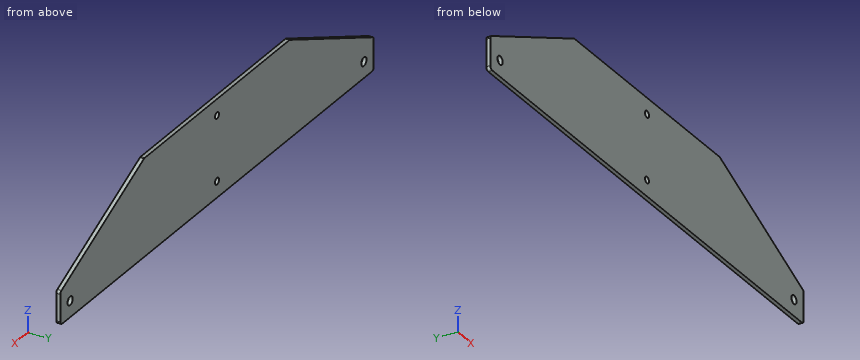
```python
from build123d import *

# Parameters (mm, degrees)
SKETCH1_W           = 406.4
SKETCH1_H           = 76.2
SKETCH1_R           = 3.3734375
SKETCH1_R_2         = 2.5796875
BOSS_EXTRUDE1_DEPTH = 3.175
CHAMFER1_SIZE       = 50.8
CHAMFER1_SIZE2      = 108.940951562
CHAMFER2_SIZE       = 50.8
CHAMFER2_SIZE2      = 108.940951562
FILLET1_R           = 2.54


with BuildPart() as part:
    # Sketch1 → Boss-Extrude1 (new body)
    with BuildSketch(Plane(origin=(0, 0, 0), x_dir=(1, 0, 0), z_dir=(0, 1, 0))):
        Rectangle(SKETCH1_W, SKETCH1_H)
        with Locations(Location((-190.5, 25.4, 0), (0, 0, 270))):
            Circle(SKETCH1_R, mode=Mode.SUBTRACT)
        with Locations(Location((190.5, 25.4, 0), (0, 0, 270))):
            Circle(SKETCH1_R, mode=Mode.SUBTRACT)
        with Locations(Location((0, 25.4, 0), (0, 0, 270))):
            Circle(SKETCH1_R_2, mode=Mode.SUBTRACT)
        with Locations(Location((0, -25.4, 0), (0, 0, 270))):
            Circle(SKETCH1_R_2, mode=Mode.SUBTRACT)
    extrude(amount=BOSS_EXTRUDE1_DEPTH)

    # Chamfer1
    chamfer1_edges = [part.edges().sort_by_distance(p)[0] for p in [
        (-203.2, 1.5875, 38.1),
    ]]
    chamfer1_side = [part.faces().sort_by_distance(p)[0] for p in [
        (-203.2, 1.5875, 0),
    ]]
    chamfer(chamfer1_edges, length=CHAMFER1_SIZE, length2=CHAMFER1_SIZE2, reference=chamfer1_side[0])

    # Chamfer2
    chamfer2_edges = [part.edges().sort_by_distance(p)[0] for p in [
        (203.2, 1.5875, 38.1),
    ]]
    chamfer2_side = [part.faces().sort_by_distance(p)[0] for p in [
        (203.2, 1.5875, 0),
    ]]
    chamfer(chamfer2_edges, length=CHAMFER2_SIZE, length2=CHAMFER2_SIZE2, reference=chamfer2_side[0])

    # Fillet1
    fillet1_edges = [part.edges().sort_by_distance(p)[0] for p in [
        (-94.259048438, 1.5875, 38.1),
        (-203.2, 1.5875, -12.7),
        (203.2, 1.5875, -12.7),
        (94.259048438, 1.5875, 38.1),
        (-203.2, 1.5875, -38.1),
        (203.2, 1.5875, -38.1),
    ]]
    fillet(fillet1_edges, radius=FILLET1_R)


solid = part.part
```
CAD build for the part. Positions are in the model's coordinates, mm. Coordinates: 2 decimals unless noted, no trailing zeros. Order: outer loops, then holes, each group sorted by start corner. A loop starts at its lowest first (then second) coordinate and runs counter-clockwise, first axis right, second up. Notation, with made-up numbers: (83, 32.25) -> (98, 32.25) arc R16 cw to (98, 54.25) -> close; hole circle Ø9 at (27.25, 51). An arc over 180 degrees is marked (long way). Use one line per item in the form item = value. Start each with the question number.
1) Drill centre lines: L1, parallel to X at y = 1.55, z = -25.4; L2, parallel to Z at x = -190.5, y = 2.2; L3, parallel to Z at x = 110.5, y = 1. Where is each one in solid material? Low to high. Write a range as [from, to].
2) Band-saw the part on A-A on y = 2.65. Give the cut face in (x, z), then the cut area to 3 significant figures.
3) Band-saw the part on B-B on x = -190.5. Give the cut face in (y, z) (3 decimals), then the cut area to 3 significant figures.
4) Band-saw the part on D-D on x = 162.5. Give the cut face in (y, z) (3 decimals), then the cut area to 3 significant figures.
5) Band-saw the part on C-C on z = -8. Give the cut face in (x, y) (3 decimals), then the cut area to 3 significant figures.
Entries:
q1.L1 = [-203.2, -193.87], [-187.13, -2.58], [2.58, 187.13], [193.87, 203.2]
q1.L2 = [-38.1, -28.77], [-22.03, -6.78]
q1.L3 = [-38.1, 30.53]
q2.outline = (-203.2, -35.56) arc R2.54 ccw to (-200.66, -38.1) -> (200.66, -38.1) arc R2.54 ccw to (203.2, -35.56) -> (203.2, -14.32) arc R2.54 ccw to (201.73, -12.02) -> (94.77, 37.86) arc R2.54 ccw to (93.7, 38.1) -> (-93.7, 38.1) arc R2.54 ccw to (-94.77, 37.86) -> (-201.73, -12.02) arc R2.54 ccw to (-203.2, -14.32) -> close; hole circle Ø6.75 at (-190.5, -25.4); hole circle Ø5.16 at (0, -25.4); hole circle Ø5.16 at (0, 25.4); hole circle Ø6.75 at (190.5, -25.4)
q2.area = 25,300 mm2
q3.outline = (0, -38.1) -> (3.175, -38.1) -> (3.175, -28.773) -> (0, -28.773) -> close; (0, -22.027) -> (3.175, -22.027) -> (3.175, -6.778) -> (0, -6.778) -> close
q3.area = 78.0 mm2
q4.outline = (0, -38.1) -> (3.175, -38.1) -> (3.175, 6.279) -> (0, 6.279) -> close
q4.area = 141 mm2
q5.outline = (-193.121, 0) -> (193.121, 0) -> (193.121, 3.175) -> (-193.121, 3.175) -> close
q5.area = 1,230 mm2
